```python
from build123d import *

# Parameters (mm, degrees)
SCHIZZO1_W                            = 150
SCHIZZO1_H                            = 30
ESTRUSIONE_ESTRUSIONE1_DEPTH          = 3
FORO_SVASATO_PER_VITE_M3_1_AT_2_COUNT = 2
FORO_SVASATO_PER_VITE_M3_1_AT_2_PITCH = 20
FORO_SVASATO_PER_VITE_M3_1_AT_3_COUNT = 2
FORO_SVASATO_PER_VITE_M3_1_AT_3_PITCH = 141.421356237
FORO_SVASATO_PER_VITE_M3_1_AT_4_COUNT = 2
FORO_SVASATO_PER_VITE_M3_1_AT_4_PITCH = 140
RACCORDO1_R                           = 5
FORO_PER_VITE_M3_1_D                  = 3.4


with BuildPart() as part:
    # Schizzo1 → Estrusione-Estrusione1 (new body)
    with BuildSketch(Plane(origin=(0, 0, 0), x_dir=(1, 0, 0), z_dir=(0, 1, 0))):
        Rectangle(SCHIZZO1_W, SCHIZZO1_H)
    extrude(amount=ESTRUSIONE_ESTRUSIONE1_DEPTH)

    # Schizzo2 → Foro svasato per Vite M3-1 (revolve, cut)
    with BuildSketch(Plane(origin=(-70, 3, -10), x_dir=(0, 0, 1), z_dir=(1, 0, 0))):
        Polygon((0, 0), (0, 3), (1.7, 3), (1.7, 1.45), (3.15, 0), align=None)
    foro_svasato_per_vite_m3_1 = revolve(axis=Axis((-70, 9.35, -10), (0, -1, 0)), mode=Mode.SUBTRACT)

    # Foro svasato per Vite M3-1 at 2: Foro svasato per Vite M3-1 ×2
    with Locations(*[(0, 0, i * FORO_SVASATO_PER_VITE_M3_1_AT_2_PITCH) for i in range(1, FORO_SVASATO_PER_VITE_M3_1_AT_2_COUNT)]):
        add(foro_svasato_per_vite_m3_1, mode=Mode.SUBTRACT)

    # Foro svasato per Vite M3-1 at 3: Foro svasato per Vite M3-1 ×2
    with Locations(*[Vector(0.9899494936611667, 0, 0.1414213562373092) * (i * FORO_SVASATO_PER_VITE_M3_1_AT_3_PITCH) for i in range(1, FORO_SVASATO_PER_VITE_M3_1_AT_3_COUNT)]):
        add(foro_svasato_per_vite_m3_1, mode=Mode.SUBTRACT)

    # Foro svasato per Vite M3-1 at 4: Foro svasato per Vite M3-1 ×2
    with Locations(*[(i * FORO_SVASATO_PER_VITE_M3_1_AT_4_PITCH, 0, 0) for i in range(1, FORO_SVASATO_PER_VITE_M3_1_AT_4_COUNT)]):
        add(foro_svasato_per_vite_m3_1, mode=Mode.SUBTRACT)

    # Raccordo1
    raccordo1_edges = [part.edges().sort_by_distance(p)[0] for p in [
        (-75, 1.5, -15),
        (75, 1.5, -15),
        (75, 1.5, 15),
        (-75, 1.5, 15),
    ]]
    fillet(raccordo1_edges, radius=RACCORDO1_R)

    # Foro per Vite M3-1 (through all)
    with Locations(Plane(origin=(0, 3, 0), x_dir=(1, 0, 0), z_dir=(0, 1, 0))):
        with Locations((17.78, -11.607048139), (-17.78, -11.607048139), (-17.78, 11.252951861), (17.78, 11.252951861)):
            Hole(FORO_PER_VITE_M3_1_D / 2)


solid = part.part
```
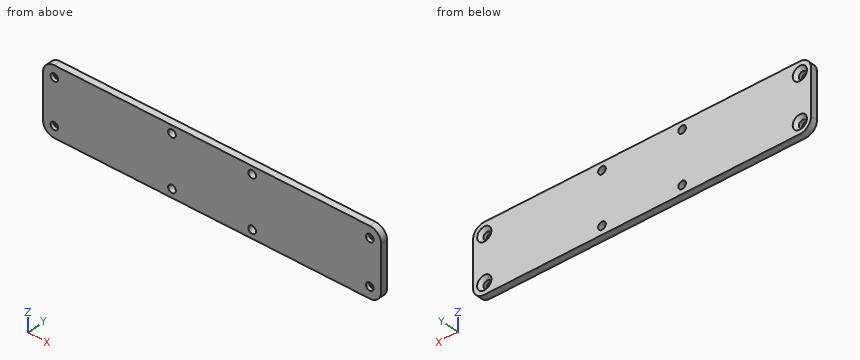
The listing builds one solid part. Answer for the finished solid, in the listing's coordinates (mm). Round coordinates to 2 decimals unless told otherwise and drop trailing zeros. Write each loop counter-clockwise with the first axis right and the second up, starting at its lowest first coordinate (ties: lowest second). Pieces come first, ordered by that corner, then holes. Notation, with made-up numbers: (-28, 11) -> (17, 11) arc R31 ccw to (17, 42) -> close; hole circle Ø10 at (-24.75, -28). An arc over 180 degrees is marked (long way). Answer as a JSON object with one key per item and string values. Group by question number.
Q1. Section B-B (y = 0.55) is taken. Count the separate pieces of the cut face and the enclosed holes in it, plus the area to 3 significant figures.
Q2. Straight lines are drawn through the part: line 1 along Z through (x, y) = (70, 1.2); line 2 along Z through (x, y) = (-17.78, 1.5); line 3 along X through (y, z) = (2.1, 8.25). For each, find the intervals that lie inside material, in ascending order.
Q3. This flat-tipped pin is pushed along its axis until it touches: pin 1 Ø4 at (x, z) = (-70, 10) entering from +Y. Where does it stop, or does it pass through?
Q4. Section A-A (x = -17.78) is taken. Write down the section's boundary in (y, z).
Check values:
{
 "1": {"separate pieces": "1", "enclosed holes": "8", "area": "4,410 mm^2"},
 "2": {"line 1": "-15 to -11.7, -8.3 to 8.3, 11.7 to 15", "line 2": "-15 to -12.95, -9.55 to 9.91, 13.31 to 15", "line 3": "-75 to -71.41, -68.59 to 68.59, 71.41 to 75"},
 "3": {"pin 1": "y = 1.85"},
 "4": {"outline": "(0, -15) -> (3, -15) -> (3, -12.95) -> (0, -12.95) -> close; (0, -9.55) -> (3, -9.55) -> (3, 9.91) -> (0, 9.91) -> close; (0, 13.31) -> (3, 13.31) -> (3, 15) -> (0, 15) -> close"}
}
